from build123d import *

# Parameters (mm, degrees)
SKETCH2_R           = 0.95
BOSS_EXTRUDE1_DEPTH = 4
SKETCH3_W           = 16.2
SKETCH3_H           = 26.26
CUT_EXTRUDE1_DEPTH  = 2


with BuildPart() as part:
    # Sketch2 → Boss-Extrude1 (new body)
    with BuildSketch(Plane.XY):
        with BuildLine():
            Line((0, 7), (0, 19.26))
            Line((0, 19.26), (4, 19.26))
            Line((4, 19.26), (4, 21.26))
            Line((4, 21.26), (0, 21.26))
            Line((0, 21.26), (0, 24.26))
            ThreePointArc((0, 24.26), (0.585786438, 25.674213562), (2, 26.26))
            Line((2, 26.26), (14.2, 26.26))
            ThreePointArc((14.2, 26.26), (15.614213562, 25.674213562), (16.2, 24.26))
            Line((16.2, 24.26), (16.2, 21.26))
            Line((16.2, 21.26), (12.2, 21.26))
            Line((12.2, 21.26), (12.2, 19.26))
            Line((12.2, 19.26), (16.2, 19.26))
            Line((16.2, 19.26), (16.2, 7))
            Line((16.2, 7), (12.2, 7))
            Line((12.2, 7), (12.2, 5))
            Line((12.2, 5), (16.2, 5))
            Line((16.2, 5), (16.2, 2))
            ThreePointArc((16.2, 2), (15.614213562, 0.585786438), (14.2, 0))
            Line((14.2, 0), (2, 0))
            ThreePointArc((2, 0), (0.585786438, 0.585786438), (0, 2))
            Line((0, 2), (0, 5))
            Line((0, 5), (4, 5))
            Line((4, 5), (4, 7))
            Line((4, 7), (0, 7))
        make_face()
        with Locations((13.45, 2.5)):
            Circle(SKETCH2_R, mode=Mode.SUBTRACT)
        with Locations((10.2, 9.5)):
            Circle(SKETCH2_R, mode=Mode.SUBTRACT)
        with Locations((2.75, 23.76)):
            Circle(SKETCH2_R, mode=Mode.SUBTRACT)
        with Locations((6, 16.76)):
            Circle(SKETCH2_R, mode=Mode.SUBTRACT)
        with Locations((10.2, 16.76)):
            Circle(SKETCH2_R, mode=Mode.SUBTRACT)
        with Locations((13.45, 23.76)):
            Circle(SKETCH2_R, mode=Mode.SUBTRACT)
        with Locations((6, 9.5)):
            Circle(SKETCH2_R, mode=Mode.SUBTRACT)
        with Locations((2.75, 2.5)):
            Circle(SKETCH2_R, mode=Mode.SUBTRACT)
    extrude(amount=BOSS_EXTRUDE1_DEPTH)

    # Sketch3 → Cut-Extrude1 (cut)
    with BuildSketch(Plane.XY.offset(4)):
        with Locations((8.1, 13.13)):
            Rectangle(SKETCH3_W, SKETCH3_H)
    extrude(amount=-CUT_EXTRUDE1_DEPTH, mode=Mode.SUBTRACT)


solid = part.part
Geometry check sheet. Reference: the model listing, model coordinates, mm. A direction names the side the tool comes from. Give positions to 0.01 mm unless a question says otherwise; leave off trailing zeros. Write each loop counter-clockwise with the first axis right and the second up, starting at its lowest first coordinate (ties: lowest second). Pieces come first, ordered by that corner, then holes.
1) Go/stop test with flat-tipped pins: pin 1 Ø1 at (y, z) = (6, 1) entering from +X; pin 2 Ø1.5 at (x, y) = (13.45, 23.76) entering from -Z; pin 3 Ø0.6 at (x, z) = (1.5, 0.5) entering from +Y. Record where each tip stops, or that it passes through.
Values follow:
pin 1: stops at x = 12.2
pin 2: passes through
pin 3: stops at y = 26.25
2) Cross-section at B-B (z = 1.2). Count the separate pieces of the cut face and the enclosed holes in it, plus the area to 3 significant figures.
Values follow:
separate pieces: 1
enclosed holes: 8
area: 367 mm2
3) Cross-section at D-D (x = 10.2). Record the boundary of the cut face in (y, z).
Values follow:
outline: (0, 0) - (8.55, 0) - (8.55, 2) - (0, 2) - close; (10.45, 0) - (15.81, 0) - (15.81, 2) - (10.45, 2) - close; (17.71, 0) - (26.26, 0) - (26.26, 2) - (17.71, 2) - close
4) Cross-section at A-A (x = 2.75). Record the boundary of the cut face in (y, z).
Values follow:
outline: (0, 0) - (1.55, 0) - (1.55, 2) - (0, 2) - close; (3.45, 0) - (5, 0) - (5, 2) - (3.45, 2) - close; (7, 0) - (19.26, 0) - (19.26, 2) - (7, 2) - close; (21.26, 0) - (22.81, 0) - (22.81, 2) - (21.26, 2) - close; (24.71, 0) - (26.26, 0) - (26.26, 2) - (24.71, 2) - close
5) Thickness scan on line 1 (X direction, y = 9.5, z = 1.4); line 2 (X direction, y = 23.76, z = 0.9); line 3 (Y direction, x = 2.75, z = 0.9). Record the ranges inside material, lowest first.
Values follow:
line 1: x = 0 to 5.05, 6.95 to 9.25, 11.15 to 16.2
line 2: x = 0 to 1.8, 3.7 to 12.5, 14.4 to 16.2
line 3: y = 0 to 1.55, 3.45 to 5, 7 to 19.26, 21.26 to 22.81, 24.71 to 26.26
6) Set-up check for faces 4 (the face through (14, 19.26, 1)), 5 (the face through (4, 20, 1)), 6 (the face through (8, 13, 2)): record each of +Z, -Z, +X, -X, +Y, -Y from which the full face is reachable in a straight line by a thin tool's end or side.
Values follow:
face 4: +Z, -Z, +X
face 5: +Z, -Z, -X
face 6: +Z, +X, -X, +Y, -Y
7) Cross-section at C-C (y = 2.5). Record the boundary of the cut face in (x, z), plus the area to 3 significant figures.
Values follow:
outline: (0, 0) - (1.8, 0) - (1.8, 2) - (0, 2) - close; (3.7, 0) - (12.5, 0) - (12.5, 2) - (3.7, 2) - close; (14.4, 0) - (16.2, 0) - (16.2, 2) - (14.4, 2) - close
area: 24.8 mm2
8) Release check for a two-part mould opening along Y. For faces 1 (the face through (15.6, 25.69, 0.99)), 2 (the face through (0, 3, 1)), 3 (the face through (14, 5, 1)) record: released by +Y, released by -Y, zero draft, split by the parting line, or undercut.
Values follow:
face 1: released by +Y
face 2: zero draft
face 3: undercut
